```python
from build123d import *

# Parameters (mm, degrees)
BASE_FLANGE1_DEPTH      = 56
SKETCH9_W               = 85
SKETCH9_H               = 21
CUT_EXTRUDE2_DEPTH      = 9
CUT_EXTRUDE3_DEPTH      = 10
SKETCH11_R              = 13
CUT_EXTRUDE4_DEPTH      = 10
BREAK_CORNER1_START     = -68
BREAK_CORNER1_DEPTH     = 5
BREAK_CORNER1_2_DEPTH   = 5
EDGE_FLANGE1_DEPTH      = 82.5
EDGE_FLANGE1_START      = -5
EDGE_FLANGE1_PROFILE_W  = 102.5
EDGE_FLANGE1_PROFILE_H  = 34
EDGE_FLANGE1_FLAT_DEPTH = 5
SKETCH15_W              = 200
SKETCH15_H              = 60
SKETCH15_R              = 7.5
BOSS_EXTRUDE1_DEPTH     = 5
BREAK_CORNER2_START     = -144.603336753
BREAK_CORNER2_OUTLINE_W = 46
BREAK_CORNER2_OUTLINE_H = 8
BREAK_CORNER2_DEPTH     = 21.213203436
BREAK_CORNER3_START     = -9
BREAK_CORNER3_DEPTH     = 5
CUT_EXTRUDE5_DEPTH      = 236.599766553
FILLET1_R               = 9


# Read off the part's stored shape, not the designer's step: Break-Corner1, Break-Corner2, Break-Corner3
# Sheet-metal steps are written as plain solids
with BuildPart() as part:
    # Sketch1 → Base-Flange1 (new body)
    with BuildSketch(Plane(origin=(0, 0, 0), x_dir=(1, 0, 0), z_dir=(0, 1, 0))):
        with BuildLine():
            Line((-63, 80), (-63, 4))
            ThreePointArc((-63, 4), (-61.828427125, 1.171572875), (-59, 0))
            Line((-59, 0), (-4, 0))
            ThreePointArc((-4, 0), (-1.171572875, 1.171572875), (0, 4))
            Line((0, 4), (0, 86.5))
            Line((0, 86.5), (5, 86.5))
            Line((5, 86.5), (5, 4))
            ThreePointArc((5, 4), (2.363961031, -2.363961031), (-4, -5))
            Line((-4, -5), (-59, -5))
            ThreePointArc((-59, -5), (-65.363961031, -2.363961031), (-68, 4))
            Line((-68, 4), (-68, 80))
            Line((-68, 80), (-63, 80))
        make_face()
    extrude(amount=BASE_FLANGE1_DEPTH)

    # Sketch9 → Cut-Extrude2 (cut)
    with BuildSketch(Plane.ZY.offset(68)):
        with Locations((-37.5, 10.5)):
            Rectangle(SKETCH9_W, SKETCH9_H)
    extrude(amount=-CUT_EXTRUDE2_DEPTH, mode=Mode.SUBTRACT)

    # Sketch10 → Cut-Extrude3 (cut)
    with BuildSketch(Plane(origin=(-63, 0, 0), x_dir=(0, 0, -1), z_dir=(1, 0, 0))):
        with BuildLine():
            Line((24.5, 44.5), (59.5, 44.5))
            ThreePointArc((59.5, 44.5), (65.5, 38.5), (59.5, 32.5))
            Line((59.5, 32.5), (24.5, 32.5))
            ThreePointArc((24.5, 32.5), (18.5, 38.5), (24.5, 44.5))
        make_face()
    extrude(amount=-CUT_EXTRUDE3_DEPTH, mode=Mode.SUBTRACT)

    # Sketch11 → Cut-Extrude4 (cut)
    with BuildSketch(Plane(origin=(5, 0, 0), x_dir=(0, 0, -1), z_dir=(1, 0, 0))):
        with Locations((51.5, 26)):
            Circle(SKETCH11_R)
    extrude(amount=-CUT_EXTRUDE4_DEPTH, mode=Mode.SUBTRACT)

    # Break-Corner1 outline → Break-Corner1 (cut)
    with BuildSketch(Plane.YZ.offset(BREAK_CORNER1_START)):
        Polygon((21, -80), (33.5, -80), (21, -67.5), align=None)
        Polygon((56, -67.5), (43.5, -80), (56, -80), align=None)
    extrude(amount=BREAK_CORNER1_DEPTH, mode=Mode.SUBTRACT)

    # Break-Corner1 2 outline → Break-Corner1 2 (cut)
    with BuildSketch(Plane.YZ):
        Polygon((56, -86.5), (56, -74), (43.5, -86.5), align=None)
    extrude(amount=BREAK_CORNER1_2_DEPTH, mode=Mode.SUBTRACT)

    # Edge-Flange1 bend section (across the edge) → Edge-Flange1 (add)
    with BuildSketch(Plane(origin=(0, -4, -86.5), x_dir=(0, 1, 0), z_dir=(0, 0, 1))):
        with BuildLine():
            Line((-5, 4), (0, 4))
            ThreePointArc((0, 4), (1.171572875, 1.171572875), (4, 0))
            Line((4, 0), (4, -5))
            ThreePointArc((4, -5), (-2.363961031, -2.363961031), (-5, 4))
        make_face()
    extrude(amount=EDGE_FLANGE1_DEPTH)

    # Edge-Flange1 profile (on flange) → Edge-Flange1 flat (add)
    with BuildSketch(Plane(origin=(0, -4, 0), x_dir=(0, 0, -1), z_dir=(0, 1, 0)).offset(EDGE_FLANGE1_START)):
        with Locations((55.25, 21)):
            Rectangle(EDGE_FLANGE1_PROFILE_W, EDGE_FLANGE1_PROFILE_H)
    extrude(amount=EDGE_FLANGE1_FLAT_DEPTH)

    # Sketch15 → Boss-Extrude1 (add)
    with BuildSketch(Plane(origin=(0, -4, 0), x_dir=(1, 0, 0), z_dir=(0, 1, 0))):
        with Locations((62, 136.5)):
            Rectangle(SKETCH15_W, SKETCH15_H)
        with Locations(Location((87, 136.5, 0), (0, 0, 180))):
            Circle(SKETCH15_R, mode=Mode.SUBTRACT)
        with Locations(Location((137, 136.5, 0), (0, 0, 180))):
            Circle(SKETCH15_R, mode=Mode.SUBTRACT)
    extrude(amount=-BOSS_EXTRUDE1_DEPTH)

    # Break-Corner2 outline → Break-Corner2 (cut)
    with BuildSketch(Plane(origin=(0, 0, 0), x_dir=(0.7071067811865471, 0, -0.707106781186548), z_dir=(0.707106781186548, 0, 0.707106781186547)).offset(BREAK_CORNER2_START)):
        with Locations((91, -7)):
            Rectangle(BREAK_CORNER2_OUTLINE_W, BREAK_CORNER2_OUTLINE_H)
    extrude(amount=BREAK_CORNER2_DEPTH, mode=Mode.SUBTRACT)

    # Break-Corner3 outline → Break-Corner3 (cut)
    with BuildSketch(Plane(origin=(0, 0, 0), x_dir=(1, 0, 0), z_dir=(0, 1, 0)).offset(BREAK_CORNER3_START)):
        Polygon((162, 106.5), (162, 118.5), (150, 106.5), align=None)
        Polygon((150, 166.5), (162, 154.5), (162, 166.5), align=None)
    extrude(amount=BREAK_CORNER3_DEPTH, mode=Mode.SUBTRACT)

    # Sketch16 → Cut-Extrude5 (cut, through all)
    with BuildSketch(Plane(origin=(5, 0, 0), x_dir=(0, 0, -1), z_dir=(1, 0, 0))):
        with BuildLine():
            Line((-5, 13.5), (-5, 0))
            Line((-5, 0), (4, 0))
            ThreePointArc((4, 0), (0.759222528, 7.589481685), (-5, 13.5))
        make_face()
    extrude(amount=-CUT_EXTRUDE5_DEPTH, mode=Mode.SUBTRACT)

    # Fillet1
    fillet1_edges = [part.edges().sort_by_distance(p)[0] for p in [
        (-4, -6.5, -106.5),
    ]]
    fillet(fillet1_edges, radius=FILLET1_R)


solid = part.part
```
Verification items for the finished model (mm, model axes). A direction names the side the tool comes from. Round coordinates to 2 decimals unless told otherwise and drop trailing zeros. Order: outer loops, then holes, each group sorted by start corner. A loop starts at its lowest first (then second) coordinate and runs counter-clockwise, first axis right, second up. Notation, with made-up numbers: (81, 11.5) -> (107, 11.5) arc R13 ccw to (107, 24.5) -> close; hole circle Ø9 at (16.5, 25). An arc over 180 degrees is marked (long way). Put each result on its own line as item: value. Start each with the question number.
(1) Material ranges on line 1 along X through (y, z) = (-5, -136); line 2 along Z through (x, y) = (87, -5.1); line 3 along X through (y, z) = (53, -27.5), recorded low to high.
(2) Tool access check on faces 1 (the face through (2, 18, -86.5)), 2 (the face through (-59, 16, 2)), 3 (the face through (-63, 30, -43)), 4 (the face through (-65.5, 38.6, -65.5)), 5 (the face through (0, 28, -36)). Record the directions out of +Z, -Z, +X, -X, +Y, -Y that give a thin tool (end or side, any length) a straight path to the whole face; none if there is none.
(3) Draft check along Y on faces 6 (the face through (-65.5, 38.4, -18.5)), 7 (the face through (-65.5, 27.3, -73.8)), 8 (the face through (-23.2, -6.5, -151.3)). Enter one of: +Y half, -Y half, draft (parallel to the pull), parting line (faces both ways), or undercut.
(4) Section check B-B (x = 137). Enter the section's corners in (y, z), then the cut area to 3 significant figures.
(5) Section check A-A (y = 26). Enter the section's corners in (x, z).
(6) Section check D-D (z = -51.5). Enter the section's corners in (x, y), then the cut area to 3 significant figures.
(7) Section check C-C (z = -13.5). Enter the section's corners in (x, y), then the cut area to 3 significant figures.
(8) Depth check by flat-ended pin: pin 1 Ø1.5 at (x, z) = (-65.5, -47) entering from -Y; pin 2 Ø17.5 at (y, z) = (45, -43) entering from +X; pin 3 Ø2.5 at (x, y) = (48.5, -7) entering from +Z. Enter the tip coordinate at first touch or a pass-through.
Completed:
1. line 1: x = -38 to 79.52, 94.48 to 129.52, 144.48 to 162
1. line 2: z = -166.5 to -144, -129 to -106.5
1. line 3: x = -68 to -63, 0 to 5
2. face 1: +X, +Y, -Y
2. face 2: +Z, -Z, -X, -Y
2. face 3: -Z, +Y, -Y
2. face 4: -X
2. face 5: -Z, +Y
3. face 6: undercut
3. face 7: -Y half
3. face 8: draft
4. outline: (-9, -166.5) -> (-4, -166.5) -> (-4, -144) -> (-9, -144) -> close; (-9, -129) -> (-4, -129) -> (-4, -106.5) -> (-9, -106.5) -> close
4. area: 225 mm2
5. outline: (-68, -72.5) -> (-63, -72.5) -> (-63, -4) arc R4 cw to (-59, 0) -> (-4, 0) arc R4 cw to (0, -4) -> (0, -38.5) -> (5, -38.5) -> (5, -4) arc R9 ccw to (-4, 5) -> (-59, 5) arc R9 ccw to (-68, -4) -> close; (0, -86.5) -> (5, -86.5) -> (5, -64.5) -> (0, -64.5) -> close
6. outline: (-68, 21) -> (-63, 21) -> (-63, 32.5) -> (-68, 32.5) -> close; (-68, 44.5) -> (-63, 44.5) -> (-63, 56) -> (-68, 56) -> close; (-38, -9) -> (-4, -9) arc R9 ccw to (5, 0) -> (5, 13) -> (0, 13) -> (0, 0) arc R4 cw to (-4, -4) -> (-38, -4) -> close; (0, 39) -> (5, 39) -> (5, 56) -> (0, 56) -> close
6. area: 486 mm2
7. outline: (-68, 21) -> (-63, 21) -> (-63, 56) -> (-68, 56) -> close; (-38, -9) -> (-4, -9) arc R9 ccw to (5, 0) -> (5, 56) -> (0, 56) -> (0, 0) arc R4 cw to (-4, -4) -> (-38, -4) -> close
7. area: 676 mm2
8. pin 1: stops at y = 21
8. pin 2: stops at x = 5
8. pin 3: stops at z = -106.5
